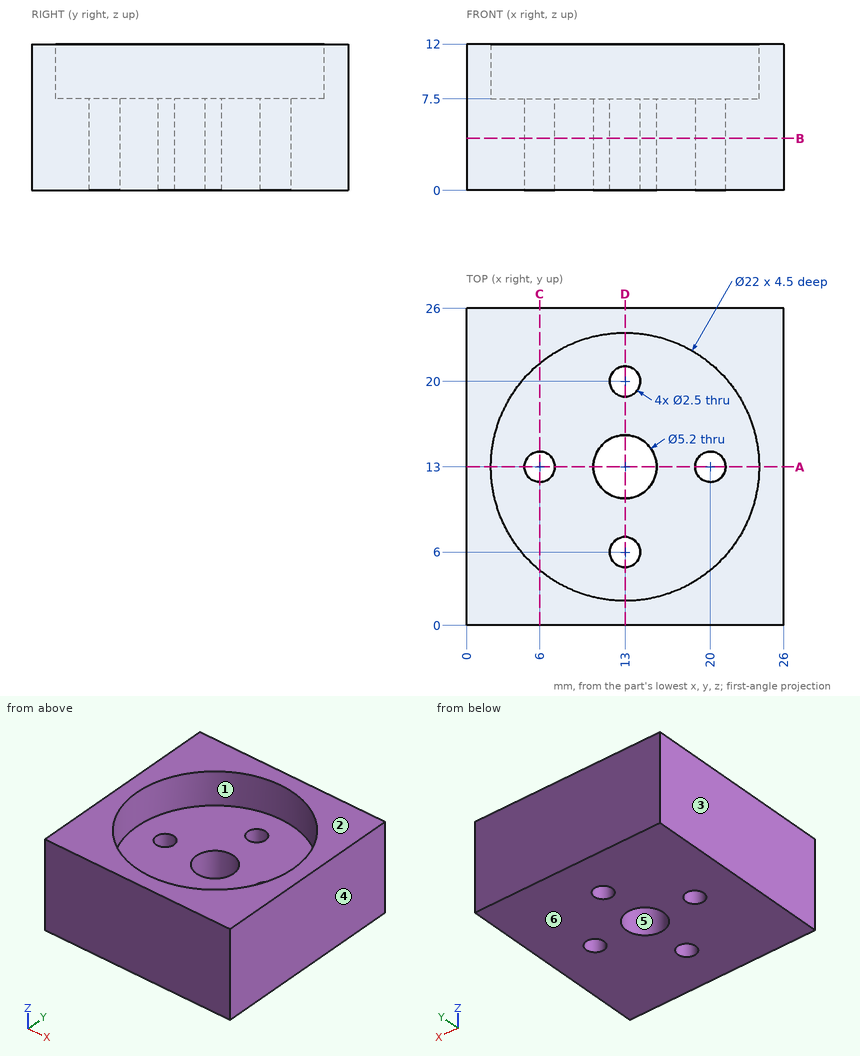
Drawing for the job (mm, zero at the part's lowest x, y, z). A direction names the side the tool comes from. Round coordinates to 2 decimals unless told otherwise and drop trailing zeros. Write each loop counter-clockwise with the first axis right and the second up, starting at its lowest first coordinate (ties: lowest second). Pieces come first, ordered by that corner, then holes. Notation, with made-up numbers: (74.25, 48.5) - (103.25, 48.5) arc R22 cw to (103.25, 83.5) - close; hole circle Ø5 at (55, 73). An arc over 180 degrees is marked (long way). Return JSON: item names as keys, results as strings. Group by question number.
Item 1: Band-saw the part on B-B on z = 4.25. List the corners of the cut face in (x, y), plus the area to 3 significant figures.
Item 2: Probe probe 1 along X at (y, z) = (13, 5.5); probe 2 along Y at (x, z) = (20, 4.75); probe 3 along Y at (x, z) = (13, 9.95). List the from-to ranges inside material, lowest first.
Item 3: Flat gauge pins, fed straight in: pin 1 Ø4 at (x, y) = (13, 20) entering from +Z; pin 2 Ø4.5 at (x, y) = (13, 13) entering from -Z. Where does each tip first touch, or does it go through?
Item 4: Band-saw the part on A-A on y = 13. List the corners of the cut face in (x, z).
Item 5: Band-saw the part on C-C on x = 6. List the corners of the cut face in (y, z), plus the area to 3 significant figures.
Item 6: Mould opens along X. For the marked faces 3, 4, 5 and 6 say: +X half, -X half, draft (parallel to the pull), parting line (faces both ways), or undercut.
Item 7: 3-axis set-ups, long thin cutter, end or side, ignore diameter. For the marked faces 1 and 2: which of +Z, -Z, +X, -X, +Y, -Y reach the whole face in a straight line?
Resolved:
{
 "1": {"outline": "(0, 0) - (26, 0) - (26, 26) - (0, 26) - close; hole circle Ø2.5 at (6, 13); hole circle Ø5.2 at (13, 13); hole circle Ø2.5 at (13, 6); hole circle Ø2.5 at (13, 20); hole circle Ø2.5 at (20, 13)", "area": "635 mm²"},
 "2": {"probe 1": "x = 0 to 4.75, 7.25 to 10.4, 15.6 to 18.75, 21.25 to 26", "probe 2": "y = 0 to 11.75, 14.25 to 26", "probe 3": "y = 0 to 2, 24 to 26"},
 "3": {"pin 1": "stops at z = 7.5", "pin 2": "passes through"},
 "4": {"outline": "(0, 0) - (4.75, 0) - (4.75, 7.5) - (2, 7.5) - (2, 12) - (0, 12) - close; (7.25, 0) - (10.4, 0) - (10.4, 7.5) - (7.25, 7.5) - close; (15.6, 0) - (18.75, 0) - (18.75, 7.5) - (15.6, 7.5) - close; (21.25, 0) - (26, 0) - (26, 12) - (24, 12) - (24, 7.5) - (21.25, 7.5) - close"},
 "5": {"outline": "(0, 0) - (11.75, 0) - (11.75, 7.5) - (4.51, 7.5) - (4.51, 12) - (0, 12) - close; (14.25, 0) - (26, 0) - (26, 12) - (21.49, 12) - (21.49, 7.5) - (14.25, 7.5) - close", "area": "217 mm²"},
 "6": {"face 3": "-X half", "face 4": "+X half", "face 5": "undercut", "face 6": "draft"},
 "7": {"face 1": "+Z", "face 2": "+Z, +X, -X, +Y, -Y"}
}
